The model under review builds one solid part; all positions refer to its coordinate system, in mm. A direction names the side the tool comes from. Coordinates: 2 decimals unless noted, no trailing zeros. Order: outer loops, then holes, each group sorted by start corner. A loop starts at its lowest first (then second) coordinate and runs counter-clockwise, first axis right, second up. Notation, with made-up numbers: (0.5, -15.75) - (27.5, -15.75) arc R17 ccw to (27.5, 15.25) - close; hole circle Ø3 at (76.25, -31.75). An arc over 180 degrees is marked (long way). Answer in a Markdown table with one row per item.
```python
from build123d import *
from build123d.topology import SkipClean

# Parameters (mm, degrees)
SKETCH1_R             = 32
SKETCH1_R_2           = 22
BOSS_EXTRUDE2_DEPTH   = 4
SKETCH3_W             = 10.5
SKETCH3_H             = 120
BOSS_EXTRUDE4_DEPTH   = 7
BOSS_EXTRUDE4_2_DEPTH = 7
BOSS_EXTRUDE5_DEPTH   = 2
SKETCH5_R             = 1.5
CUT_EXTRUDE1_DEPTH    = 4
SKETCH6_R             = 2
CUT_EXTRUDE2_DEPTH    = 4


with BuildPart() as part:
    # Sketch1 → Boss-Extrude2 (new body)
    with BuildSketch(Plane(origin=(0, 0, 0), x_dir=(1, 0, 0), z_dir=(0, 1, 0))):
        with Locations(Location((0, 0, 0), (0, 0, 270))):
            Circle(SKETCH1_R)
        with Locations(Location((0, 0, 0), (0, 0, 270))):
            Circle(SKETCH1_R_2, mode=Mode.SUBTRACT)
    extrude(amount=BOSS_EXTRUDE2_DEPTH)



with BuildPart() as body_2:
    # Sketch3 → Boss-Extrude4 (new body)
    with BuildSketch(Plane(origin=(0, 0, 0), x_dir=(1, 0, 0), z_dir=(0, 1, 0))):
        with Locations((-59.75, 0)):
            Rectangle(SKETCH3_W, SKETCH3_H)
    extrude(amount=BOSS_EXTRUDE4_DEPTH)


with BuildPart() as body_3:
    # Sketch3 → Boss-Extrude4 2 (new body)
    with BuildSketch(Plane(origin=(0, 0, 0), x_dir=(1, 0, 0), z_dir=(0, 1, 0))):
        with Locations((59.75, 0)):
            Rectangle(SKETCH3_W, SKETCH3_H)
    extrude(amount=BOSS_EXTRUDE4_2_DEPTH)


with BuildPart() as part_1:
    with SkipClean():  # the faces are left unmerged after this step: merging them gives an invalid solid
        add(part.part)

        add(body_2.part)  # Boss-Extrude5 merges body 2

        add(body_3.part)  # Boss-Extrude5 merges body 3
        # Sketch4 → Boss-Extrude5 (add)
        with BuildSketch(Plane(origin=(0, 0, 0), x_dir=(1, 0, 0), z_dir=(0, 1, 0))):
            with BuildLine():
                Line((-54.5, 50), (-42.5, 50))
                Line((-42.5, 50), (-20.316435899, 27.780252561))
                ThreePointArc((-20.316435899, 27.780252561), (-18.551903635, 26.921342904), (-16.633954414, 27.336999845))
                ThreePointArc((-16.633954414, 27.336999845), (0, 32), (16.633954414, 27.336999845))
                ThreePointArc((16.633954414, 27.336999845), (18.551903635, 26.921342904), (20.316435899, 27.780252561))
                Line((20.316435899, 27.780252561), (42.5, 50))
                Line((42.5, 50), (54.5, 50))
                Line((54.5, 50), (54.5, -50))
                Line((54.5, -50), (42.5, -50))
                Line((42.5, -50), (20.316435899, -27.780252561))
                ThreePointArc((20.316435899, -27.780252561), (18.551903635, -26.921342904), (16.633954414, -27.336999845))
                ThreePointArc((16.633954414, -27.336999845), (0, -32), (-16.633954414, -27.336999845))
                ThreePointArc((-16.633954414, -27.336999845), (-18.551903635, -26.921342904), (-20.316435899, -27.780252561))
                Line((-20.316435899, -27.780252561), (-42.5, -50))
                Line((-42.5, -50), (-54.5, -50))
                Line((-54.5, -50), (-54.5, 50))
            make_face()
            with BuildLine():
                Line((-52, -37.403142366), (-52, 37.403142366))
                ThreePointArc((-52, 37.403142366), (-50.146920927, 40.175248495), (-46.876951741, 39.522733386))
                Line((-46.876951741, 39.522733386), (-27.747104804, 20.361683992))
                ThreePointArc((-27.747104804, 20.361683992), (-26.891072048, 18.595754257), (-27.309854229, 16.678485003))
                ThreePointArc((-27.309854229, 16.678485003), (-32, 0), (-27.309854229, -16.678485003))
                ThreePointArc((-27.309854229, -16.678485003), (-26.891072048, -18.595754257), (-27.747104804, -20.361683992))
                Line((-27.747104804, -20.361683992), (-46.876951741, -39.522733386))
                ThreePointArc((-46.876951741, -39.522733386), (-50.146920927, -40.175248495), (-52, -37.403142366))
            make_face(mode=Mode.SUBTRACT)
            with BuildLine():
                Line((52, -37.403142366), (52, 37.403142366))
                ThreePointArc((52, 37.403142366), (50.146920927, 40.175248495), (46.876951741, 39.522733386))
                Line((46.876951741, 39.522733386), (27.747104804, 20.361683992))
                ThreePointArc((27.747104804, 20.361683992), (26.891072048, 18.595754257), (27.309854229, 16.678485003))
                ThreePointArc((27.309854229, 16.678485003), (32, 0), (27.309854229, -16.678485003))
                ThreePointArc((27.309854229, -16.678485003), (26.891072048, -18.595754257), (27.747104804, -20.361683992))
                Line((27.747104804, -20.361683992), (46.876951741, -39.522733386))
                ThreePointArc((46.876951741, -39.522733386), (50.146920927, -40.175248495), (52, -37.403142366))
            make_face(mode=Mode.SUBTRACT)
            with BuildLine():
                Line((-8.829338029, -1.41306068), (-16.884830668, -9.481692534))
                ThreePointArc((-16.884830668, -9.481692534), (-18.667420028, -10.034629474), (-20.130215791, -8.875495039))
                ThreePointArc((-20.130215791, -8.875495039), (-22, 0), (-20.130215791, 8.875495039))
                ThreePointArc((-20.130215791, 8.875495039), (-18.667420028, 10.034629474), (-16.884830668, 9.481692534))
                Line((-16.884830668, 9.481692534), (-8.829338029, 1.41306068))
                ThreePointArc((-8.829338029, 1.41306068), (-8.244703535, 0), (-8.829338029, -1.41306068))
            make_face(mode=Mode.SUBTRACT)
            with BuildLine():
                Line((8.829338029, -1.41306068), (16.884830668, -9.481692534))
                ThreePointArc((16.884830668, -9.481692534), (18.667420028, -10.034629474), (20.130215791, -8.875495039))
                ThreePointArc((20.130215791, -8.875495039), (22, 0), (20.130215791, 8.875495039))
                ThreePointArc((20.130215791, 8.875495039), (18.667420028, 10.034629474), (16.884830668, 9.481692534))
                Line((16.884830668, 9.481692534), (8.829338029, 1.41306068))
                ThreePointArc((8.829338029, 1.41306068), (8.244703535, 0), (8.829338029, -1.41306068))
            make_face(mode=Mode.SUBTRACT)
            with BuildLine():
                Line((-9.454161763, 16.900261103), (-1.415365506, 8.848352865))
                ThreePointArc((-1.415365506, 8.848352865), (0, 8.261413545), (1.415365506, 8.848352865))
                Line((1.415365506, 8.848352865), (9.454161763, 16.900261103))
                ThreePointArc((9.454161763, 16.900261103), (10.00419278, 18.683749248), (8.842675883, 20.144653962))
                ThreePointArc((8.842675883, 20.144653962), (0, 22), (-8.842675883, 20.144653962))
                ThreePointArc((-8.842675883, 20.144653962), (-10.00419278, 18.683749248), (-9.454161763, 16.900261103))
            make_face(mode=Mode.SUBTRACT)
            with BuildLine():
                Line((9.454161763, -16.900261103), (1.415365506, -8.848352865))
                ThreePointArc((1.415365506, -8.848352865), (0, -8.261413545), (-1.415365506, -8.848352865))
                Line((-1.415365506, -8.848352865), (-9.454161763, -16.900261103))
                ThreePointArc((-9.454161763, -16.900261103), (-10.00419278, -18.683749248), (-8.842675883, -20.144653962))
                ThreePointArc((-8.842675883, -20.144653962), (0, -22), (8.842675883, -20.144653962))
                ThreePointArc((8.842675883, -20.144653962), (10.00419278, -18.683749248), (9.454161763, -16.900261103))
            make_face(mode=Mode.SUBTRACT)
        extrude(amount=BOSS_EXTRUDE5_DEPTH)

    # Sketch5 → Cut-Extrude1 (cut)
    with SkipClean():  # the faces are left unmerged after this step: merging them gives an invalid solid
        with BuildSketch(Plane(origin=(0, 2, 0), x_dir=(1, 0, 0), z_dir=(0, 1, 0))):
            with Locations(Location((0, 0, 0), (0, 0, 270))):
                Circle(SKETCH5_R)
        extrude(amount=-CUT_EXTRUDE1_DEPTH, mode=Mode.SUBTRACT)

    # Sketch6 → Cut-Extrude2 (cut)
    with SkipClean():  # the faces are left unmerged after this step: merging them gives an invalid solid
        with BuildSketch(Plane.XZ):
            with Locations(Location((-17.309993329, -17.338227446, 0), (0, 0, 270))):
                Circle(SKETCH6_R)
            with Locations(Location((17.309993329, -17.338227446, 0), (0, 0, 270))):
                Circle(SKETCH6_R)
            with Locations(Location((17.309993329, 17.338227446, 0), (0, 0, 270))):
                Circle(SKETCH6_R)
            with Locations(Location((-17.309993329, 17.338227446, 0), (0, 0, 270))):
                Circle(SKETCH6_R)
        extrude(amount=-CUT_EXTRUDE2_DEPTH, mode=Mode.SUBTRACT)


solid = part_1.part
```
Item 1: We need section B-B, the plane z = 42.5. Write out the cut boundary in (x, y), then the cut area to 3 significant figures.
Check values:
| item | result |
|---|---|
| outline | (-65, 0) - (-35.01, 0) - (-35.01, 2) - (-54.5, 2) - (-54.5, 7) - (-65, 7) - close; (35.01, 0) - (65, 0) - (65, 7) - (54.5, 7) - (54.5, 2) - (35.01, 2) - close |
| area | 225 mm^2 |
Item 2: Tool access review of faces 1 (the face through (-21, 4, -8)), 2 (the face through (50.101, 0.986, 40.194)), 3 (the face through (-65, 3, 1)): name each direction out of +Z, -Z, +X, -X, +Y, -Y from which nothing blocks a thin tool from reaching the whole face with its end or side.
Check values:
| item | result |
|---|---|
| face 1 | +Z, -Z, +Y |
| face 2 | +Y, -Y |
| face 3 | +Z, -Z, -X, +Y, -Y |
Item 3: We need section C-C, the plane x = -13.5. Write out the cut boundary in (y, z).
Check values:
| item | result |
|---|---|
| outline | (0, -29.01) - (4, -29.01) - (4, -17.37) - (2, -17.37) - (2, -6.09) - (0, -6.09) - close; (0, 6.09) - (2, 6.09) - (2, 17.37) - (4, 17.37) - (4, 29.01) - (0, 29.01) - close |
Item 4: We need section D-D, the plane x = 50. Write out the cut boundary in (y, z).
Check values:
| item | result |
|---|---|
| outline | (0, -50) - (2, -50) - (2, -40.23) - (0, -40.23) - close; (0, 40.23) - (2, 40.23) - (2, 50) - (0, 50) - close |
Item 5: We need section A-A, the plane y = 5.5. Write out the cut boundary in (x, z).
Check values:
| item | result |
|---|---|
| outline | (-65, -60) - (-54.5, -60) - (-54.5, 60) - (-65, 60) - close; (54.5, -60) - (65, -60) - (65, 60) - (54.5, 60) - close |
Item 6: Clearance check with flat-ended pins moving along their axes: pin 1 Ø0.6 at (x, y) = (-49.5, 1) entering from -Z; pin 2 Ø19 at (x, z) = (44.5, 6.5) entering from +Y; pin 3 Ø2 at (x, y) = (45.5, 1) entering from +Z. State where each tip first meets the part, or that it passes through.
Check values:
| item | result |
|---|---|
| pin 1 | z = -50 |
| pin 2 | y = 2 |
| pin 3 | z = 50 |
Item 7: To check wall thickness, follow line 1 (X direction, y = 5, z = 28.5); line 2 (Z direction, x = 9.5, y = 1.5); line 3 (X direction, y = 1.25, z = 29.5). State the ranges of each line that lie inside material, in increasing order. Write a range as from..to.
Check values:
| item | result |
|---|---|
| line 1 | -65..-54.5, 54.5..65 |
| line 2 | -30.56..-19.68, -16.95..-2.08, 2.08..16.95, 19.68..30.56 |
| line 3 | -65..-52, -36.87..-22.03, -12.4..12.4, 22.03..36.87, 52..65 |
Item 8: Mouldability with a two-part tool opening along Z and no side actions: class faces 4 (the face through (-60, 3, 60)), 5 (the face through (-60, 7, -1)), 6 (the face through (-4, 2, 0)) as +Z half, -Z half, draft (parallel to the pull), parting line (faces both ways), or undercut.
Check values:
| item | result |
|---|---|
| face 4 | +Z half |
| face 5 | draft |
| face 6 | undercut |
